Verification items for the finished model (mm, model axes). Face numbers are marked on the shaded views. A direction names the side the tool comes from. Round coordinates to 2 decimals unless told otherwise and drop trailing zeros. Write each loop counter-clockwise with the first axis right and the second up, starting at its lowest first coordinate (ties: lowest second). Pieces come first, ordered by that corner, then holes. Notation, with made-up numbers: M 9,52.25 L 32,52.25 A18 ccw 32,57.25 Z; hole C -25.5,5.25 d3. An arc over 180 degrees is marked long. Answer in a Markdown table with one row per item. Add a question column.
1. Sectioned sample at A-A on x = 0. Record the cut outline in (y, z) (3 decimals), plus the area to 3 significant figures.
2. Sectioned sample at B-B on z = -0.75. Record the cut outline in (x, y), plus the area to 3 significant figures.
3. Draft check along Z on the marked faces 1, 2 and 3. Enter one of: pulls with the +Z half, pulls with the -Z half, needs draft (parallel to the pull), parting line crosses it, or undercut.
4. Set-up check for the marked faces 4 and 5: record each of +Z, -Z, +X, -X, +Y, -Y from which the full face is reachable in a straight line by a thin tool's end or side.
5. Go/stop test with a flat-tipped pin: pin 1 Ø1.5 at (y, z) = (4.5, -1.5) entering from -X. Record where the tip stops, or that it passes through.
6. Sectioned sample at D-D on z = 1.75. Record the cut outline in (x, y), plus the area to 3 significant figures.
7. Material ranges on probe 1 along Z at (x, y) = (1, 2.5); probe 2 along Y at (x, z) = (0, -2.75); probe 3 along Z at (x, y) = (0, 2.75), recorded low to high.
8. Sectioned sample at C-C on x = 1.75. Record the cut outline in (y, z).
Autodesk Inventor part; units mm, degrees
ref_plane "YZ Plane" through (0, 0, 0) normal (1, 0, 0) x (0, 1, 0)
ref_plane "XZ Plane" through (0, 0, 0) normal (0, 1, 0) x (-1, 0, 0)
ref_plane "XY Plane" through (0, 0, 0) normal (0, 0, 1) x (1, 0, 0)
sketch "Sketch1" plane through (0, 0, 0) normal (0, 1, 0) x (-1, 0, 0)
  circle A0 centre (0, 0) radius 3.57
  dimension "d0" = 7.14
extrude "Extrusion1" add sketch "Sketch1" along normal blind 5.35
sketch "Sketch2" plane through (0, 0, 0) normal (0, -1, 0) x (1, 0, 0)
  circle A0 centre (0, 0) radius 2.705
  dimension "d3" = 5.41
extrude "Extrusion2" add sketch "Sketch2" along normal blind 1.52
sketch "Sketch3" plane through (0, -1.52, 0) normal (0, -1, 0) x (1, 0, 0)
  point P0 (0, 0)
  point P1 (-0.1828, -0.1859)
hole "Hole1" at (-0.1828, -1.52, -0.1859) direction (0, 1, 0) diameter 2.6416 end through all
properties part number "spacer"
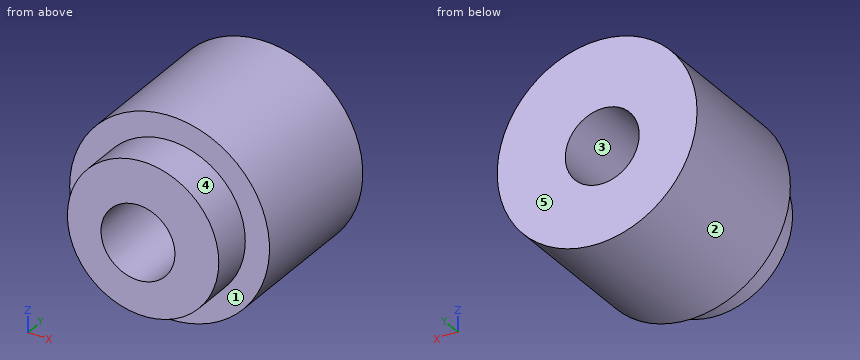
Geometry check:
| question | item | result |
|---|---|---|
| 1 | outline | M -1.52,-2.705 L 0,-2.705 L 0,-3.57 L 5.35,-3.57 L 5.35,-1.494 L -1.52,-1.494 Z; M -1.52,1.122 L 5.35,1.122 L 5.35,3.57 L 0,3.57 L 0,2.705 L -1.52,2.705 Z |
| 1 | area | 28.4 mm2 |
| 2 | outline | M -3.49,0 L -2.6,0 L -2.6,-1.52 L -1.38,-1.52 L -1.38,5.35 L -3.49,5.35 Z; M 1.01,-1.52 L 2.6,-1.52 L 2.6,0 L 3.49,0 L 3.49,5.35 L 1.01,5.35 Z |
| 2 | area | 28.8 mm2 |
| 3 | face 1 | needs draft |
| 3 | face 2 | parting line crosses it |
| 3 | face 3 | undercut |
| 4 | face 4 | -Y |
| 4 | face 5 | +Z, -Z, +X, -X, +Y |
| 5 | pin 1 | stops at x = -3.49 |
| 6 | outline | M -3.11,0 L -2.06,0 L -2.06,-1.52 L 2.06,-1.52 L 2.06,0 L 3.11,0 L 3.11,5.35 L -3.11,5.35 Z |
| 6 | area | 39.6 mm2 |
| 7 | probe 1 | z = -3.43 to -0.77, 0.4 to 3.43 |
| 7 | probe 2 | y = 0 to 5.35 |
| 7 | probe 3 | z = -3.57 to -1.49, 1.12 to 3.57 |
| 8 | outline | M -1.52,-2.06 L 0,-2.06 L 0,-3.11 L 5.35,-3.11 L 5.35,3.11 L 0,3.11 L 0,2.06 L -1.52,2.06 Z |
